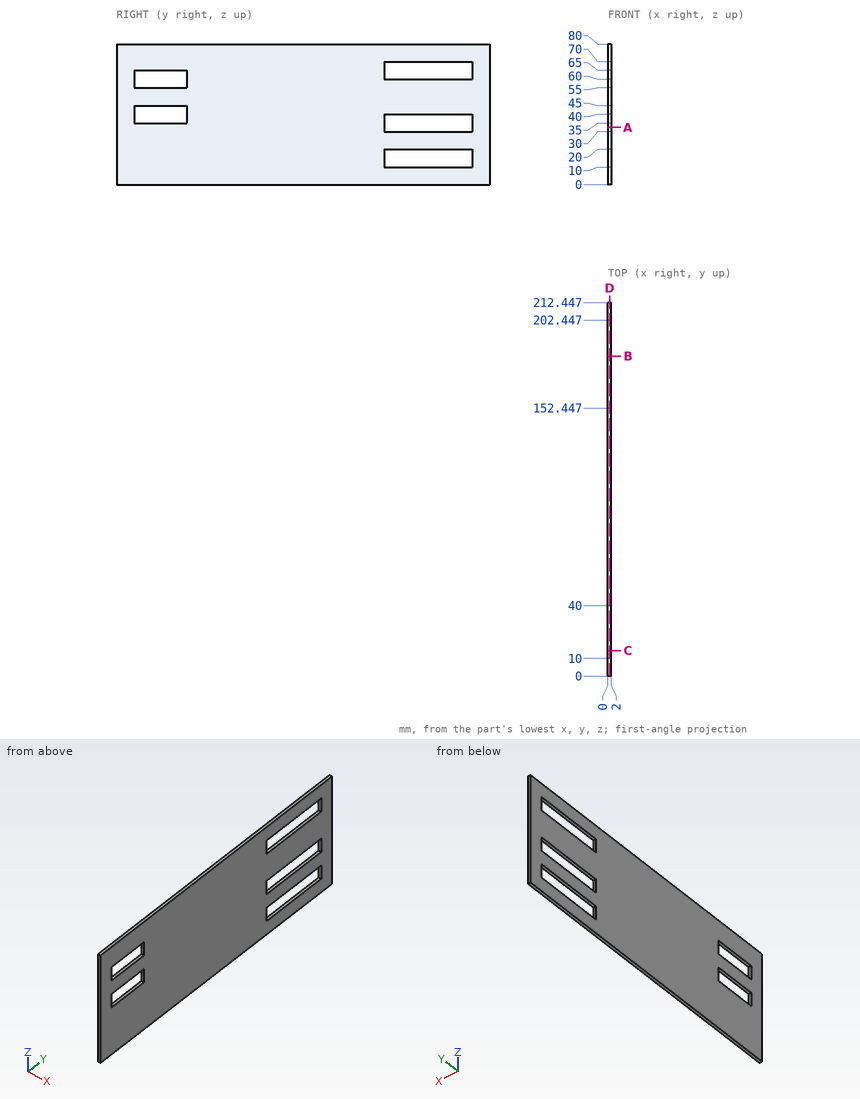
Input: dimensioned drawing with shaded views. Units: mm. Origin: part minimum x, y, z. Coordinates: 2 decimals unless noted, no trailing zeros. Write each loop counter-clockwise with the first axis right and the second up, starting at its lowest first coordinate (ties: lowest second). Pieces come first, ordered by that corner, then holes. Notation, with made-up numbers: M 62,81.5 L 107,81.5 A23 ccw 107,110.5 Z; hole C 26.5,-0.75 d10. An arc over 180 degrees is marked long. Answer as CSV lines item,"result". Start each with the question number.
Q1. Cut plane D-D on x = 1. Return the cut outline in (y, z), then the cut area to 3 significant figures.
Q2. Cut plane B-B on y = 182. Return the cut outline in (x, z).
Q3. Cut plane A-A on z = 32.5. Return the cut outline in (x, y), then the cut area to 3 significant figures.
Q4. Line query: line 1 (Z direction, x = 0.8, y = 34); line 2 (Z direction, x = 1.05, y = 185.5); line 3 (Y direction, x = 1.55, z = 61). Output: solid intervals per line, ascending. Write a range as from..to.
Q5. Cut plane C-C on y = 14.5. Return the cut outline in (x, z).
Findings below:
1,outline,"M 0,0 L 212.45,0 L 212.45,80 L 0,80 Z; hole M 10,35 L 40,35 L 40,45 L 10,45 Z; hole M 10,55 L 40,55 L 40,65 L 10,65 Z; hole M 152.45,10 L 202.45,10 L 202.45,20 L 152.45,20 Z; hole M 152.45,30 L 202.45,30 L 202.45,40 L 152.45,40 Z; hole M 152.45,60 L 202.45,60 L 202.45,70 L 152.45,70 Z"
1,area,"14,900 mm2"
2,outline,"M 0,0 L 2,0 L 2,10 L 0,10 Z; M 0,20 L 2,20 L 2,30 L 0,30 Z; M 0,40 L 2,40 L 2,60 L 0,60 Z; M 0,70 L 2,70 L 2,80 L 0,80 Z"
3,outline,"M 0,0 L 2,0 L 2,152.45 L 0,152.45 Z; M 0,202.45 L 2,202.45 L 2,212.45 L 0,212.45 Z"
3,area,"325 mm2"
4,line 1,"z = 0..35, 45..55, 65..80"
4,line 2,"z = 0..10, 20..30, 40..60, 70..80"
4,line 3,"y = 0..10, 40..152.45, 202.45..212.45"
5,outline,"M 0,0 L 2,0 L 2,35 L 0,35 Z; M 0,45 L 2,45 L 2,55 L 0,55 Z; M 0,65 L 2,65 L 2,80 L 0,80 Z"
